from build123d import *

# Parameters (mm, degrees)
SKETCH2_R           = 3.175
BOSS_EXTRUDE1_DEPTH = 1.5875


with BuildPart() as part:
    # Sketch2 → Boss-Extrude1 (new body)
    with BuildSketch(Plane.XY):
        with BuildLine():
            Line((19.05, 22.900962235), (29.734882516, 8.976152235))
            ThreePointArc((29.734882516, 8.976152235), (31.75, 7.982406265), (33.765117484, 8.976152235))
            Line((33.765117484, 8.976152235), (44.45, 22.900962235))
            Line((44.45, 22.900962235), (48.26, 22.900962235))
            ThreePointArc((48.26, 22.900962235), (50.056051224, 22.157013459), (50.8, 20.360962235))
            Line((50.8, 20.360962235), (50.8, 2.54))
            ThreePointArc((50.8, 2.54), (50.056051224, 0.743948776), (48.26, 0))
            Line((48.26, 0), (2.54, 0))
            ThreePointArc((2.54, 0), (0.743948776, 0.743948776), (0, 2.54))
            Line((0, 2.54), (0, 20.360962235))
            ThreePointArc((0, 20.360962235), (0.743948776, 22.157013459), (2.54, 22.900962235))
            Line((2.54, 22.900962235), (19.05, 22.900962235))
        make_face()
        with Locations((5.08, 17.820962235)):
            Circle(SKETCH2_R, mode=Mode.SUBTRACT)
        with Locations((5.08, 5.08)):
            Circle(SKETCH2_R, mode=Mode.SUBTRACT)
    extrude(amount=BOSS_EXTRUDE1_DEPTH)


solid = part.part
Input: part model. Units: mm. Frame: model coordinates. A direction names the side the tool comes from. Round coordinates to 2 decimals unless told otherwise and drop trailing zeros. Write each loop counter-clockwise with the first axis right and the second up, starting at its lowest first coordinate (ties: lowest second). Pieces come first, ordered by that corner, then holes.
1) Cut plane A-A (y = 5.08). Return the cut outline in (x, z) (1 decimal).
2) Ray query, L1, parallel to Y at x = 5.08, z = 1.05 (3 decimals); L2, parallel to X at y = 5, z = 1.05; L3, parallel to Y at x = 5.5, z = 0.1. Return the intervals inside material, ascending.
3) Reachability of faces 1 (the cylindrical face through (4.39, 1.98, 0.78)), 2 (the flat face through (39, 15.8, 0.8)) from +Z, -Z, +X, -X, +Y, -Y: full face, straight path, thin tool, end or side. Return the list, or none.
4) Cut plane B-B (x = 5.08). Return the cut outline in (y, z) (1 decimal), then the cut area to 3 significant figures.
5) Cut plane C-C (y = 17). Return the cut outline in (x, z).
6) Draft query along X for faces 3 (the cylindrical face through (31.717, 7.983, 0.783)), 4 (the cylindrical face through (50.036, 22.177, 0.783)), 5 (the flat face through (26, 0, 1)). Return one class per face: pulls with the +X half, pulls with the -X half, needs draft (parallel to the pull), parting line crosses it, or undercut.
7) Cut plane D-D (z = 0.6). Return the cut outline in (x, y) (3 decimals), then the cut area to 3 significant figures.
Geometry says:
1. outline: (0, 0) - (1.9, 0) - (1.9, 1.6) - (0, 1.6) - close; (8.3, 0) - (50.8, 0) - (50.8, 1.6) - (8.3, 1.6) - close
2. L1: y = 0 to 1.905, 8.255 to 14.646, 20.996 to 22.901
2. L2: x = 0 to 1.91, 8.25 to 50.8
2. L3: y = 0 to 1.93, 8.23 to 14.67, 20.97 to 22.9
3. face 1: +Z, -Z
3. face 2: +Z, -Z, +Y
4. outline: (0, 0) - (1.9, 0) - (1.9, 1.6) - (0, 1.6) - close; (8.3, 0) - (14.6, 0) - (14.6, 1.6) - (8.3, 1.6) - close; (21, 0) - (22.9, 0) - (22.9, 1.6) - (21, 1.6) - close
4. area: 16.2 mm2
5. outline: (0, 0) - (2.01, 0) - (2.01, 1.59) - (0, 1.59) - close; (8.15, 0) - (23.58, 0) - (23.58, 1.59) - (8.15, 1.59) - close; (39.92, 0) - (50.8, 0) - (50.8, 1.59) - (39.92, 1.59) - close
6. face 3: undercut
6. face 4: pulls with the +X half
6. face 5: needs draft
7. outline: (0, 2.54) arc R2.54 ccw to (2.54, 0) - (48.26, 0) arc R2.54 ccw to (50.8, 2.54) - (50.8, 20.361) arc R2.54 ccw to (48.26, 22.901) - (44.45, 22.901) - (33.765, 8.976) arc R2.54 cw to (29.735, 8.976) - (19.05, 22.901) - (2.54, 22.901) arc R2.54 ccw to (0, 20.361) - close; hole circle Ø6.35 at (5.08, 5.08); hole circle Ø6.35 at (5.08, 17.821)
7. area: 887 mm2
